Check sheet for the modelled part. Datum: model origin and axes. Units: mm. Round coordinates to 2 decimals unless told otherwise and drop trailing zeros. Write each loop counter-clockwise with the first axis right and the second up, starting at its lowest first coordinate (ties: lowest second). Pieces come first, ordered by that corner, then holes. Notation, with made-up numbers: (-15.5, 9.25) -> (6.5, 9.25) arc R14 cw to (6.5, 34.25) -> close; hole circle Ø3 at (-37.75, 83.5). An arc over 180 degrees is marked (long way). One line per item, written item: value.
Autodesk Inventor part; units mm, degrees
ref_plane "Work Plane1" through (0, 92.5, 0) normal (0, 1, 0) x (-1, 0, 0)
ref_plane "Work Plane2" through (0, 98.5, 0) normal (0, 1, 0) x (-1, 0, 0)
ref_plane "YZ Plane" through (0, 0, 0) normal (1, 0, 0) x (0, 1, 0)
sketch "Sketch1" plane through (0, 0, 0) normal (0, 1, 0) x (-1, 0, 0)
  circle A0 centre (0, 0) radius 23.5
  dimension "d0" = 47
ref_plane "Work Plane1" through (0, 92.5, 0) normal (0, 1, 0) x (-1, 0, 0)
sketch "Sketch2" plane through (0, 92.5, 0) normal (0, 1, 0) x (-1, 0, 0)
  circle A0 centre (0, 0) radius 31.375
  dimension "d2" = 62.75
ref_plane "Work Plane2" through (0, 98.5, 0) normal (0, 1, 0) x (-1, 0, 0)
sketch "Sketch3" plane through (0, 98.5, 0) normal (0, 1, 0) x (-1, 0, 0)
  circle A0 centre (0, 0) radius 35
  dimension "d4" = 70
loft "Loft1" add profiles "Sketch1", "Sketch2"
loft "Loft2" add profiles "Sketch3" section 1 edges at (31.375, 92.5, 0)
shell "Shell1" thickness 2 removed faces 1 at (1.9985, 98.5, 11.019)
properties part number "Cup_Dispenser_Cup"
Item 1: Thickness scan on line 1 (Y direction, x = 7, z = -8); line 2 (X direction, y = 61.5, z = -24); line 3 (X direction, y = 90.5, z = 6.5). Record the ranges inside material, lowest first.
Answer:
line 1: y = 0 to 2
line 2: x = -15.8 to -11.77, 11.77 to 15.8
line 3: x = -30.52 to -28.46, 28.46 to 30.52
Item 2: Mould release check, pull along Z, two halves, no side actions. Record for faces 1 (the flat face through (0, 2, 0)), 2 (the conical face through (5.96, 46.9, -26.84)), 3 (the flat face through (29, 98.5, 16)): pulls with the +Z half, pulls with the -Z half, needs draft (parallel to the pull), parting line crosses it, or undercut.
Answer:
face 1: undercut
face 2: parting line crosses it
face 3: needs draft
Item 3: Depth check by flat-ended pin: P1, Ø10, axis at x = 25.5, y = 29, coming from the +Z side; P2, Ø3, axis at y = 57.5, z = -14.5, coming from the -X side; P3, Ø13, axis at x = 5.5, z = 0, coming from the +Y side. Enter the tip coordinate at first touch or a pass-through.
Answer:
P1: stops at z = 15.98
P2: stops at x = -25.26
P3: stops at y = 2
Item 4: Sectioned sample at A-A on x = 0. Enter the section's corners in (y, z) (3 decimals).
Answer:
outline: (0, -23.5) -> (92.5, -31.375) -> (98.5, -35) -> (98.5, -32.663) -> (93.135, -29.422) -> (2, -21.663) -> (2, 21.663) -> (93.135, 29.422) -> (98.5, 32.663) -> (98.5, 35) -> (92.5, 31.375) -> (0, 23.5) -> close
Item 5: Sectioned sample at B-B on y = 33.5. Enter the section's corners in (x, z).
Answer:
outline: circle Ø52.7 at (0, 0); hole circle Ø48.69 at (0, 0)
Item 6: Sectioned sample at C-C on y = 82. Enter the section's corners in (x, z), and give its area (3 significant figures).
Answer:
outline: circle Ø60.96 at (0, 0); hole circle Ø56.95 at (0, 0)
area: 372 mm^2
